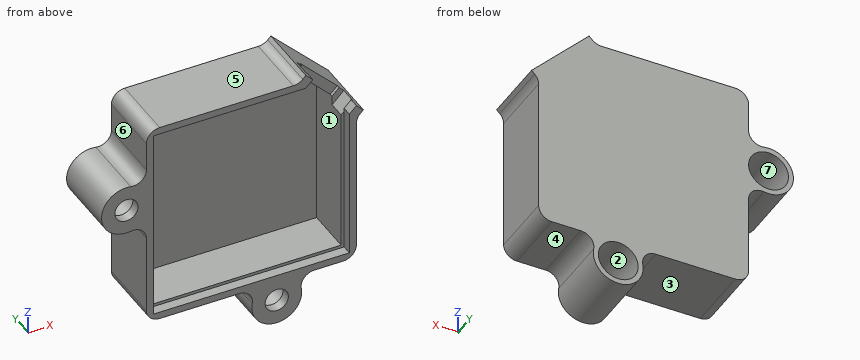
```python
from build123d import *

# Parameters (mm, degrees)
SKETCH1_W           = 31.6
SKETCH1_H           = 31.6
SKETCH1_W_2         = 28.6
SKETCH1_H_2         = 28.6
BOSS_EXTRUDE1_DEPTH = 10
SKETCH2_W           = 31.6
SKETCH2_H           = 31.6
BOSS_EXTRUDE2_DEPTH = 1.5
FILLET2_R           = 2
SKETCH3_R           = 3.75
SKETCH3_R_2         = 1.75
BOSS_EXTRUDE3_DEPTH = 10
SKETCH4_R           = 3
CUT_EXTRUDE1_DEPTH  = 8.5
CUT_EXTRUDE2_REACH  = 35.43
SKETCH6_W           = 29.5
SKETCH6_H           = 29.5
CUT_EXTRUDE3_DEPTH  = 1.5
FILLET3_R           = 2
BOSS_EXTRUDE4_DEPTH = 5.4
BOSS_EXTRUDE5_DEPTH = 4.6
BOSS_EXTRUDE6_DEPTH = 3.1
FILLET4_R           = 2
CUT_EXTRUDE6_START  = -2.5
SKETCH12_W          = 10
SKETCH12_H          = 2.6
CUT_EXTRUDE6_DEPTH  = 2.5


with BuildPart() as part:
    # Sketch1 → Boss-Extrude1 (new body)
    with BuildSketch(Plane(origin=(0, 0, 0), x_dir=(1, 0, 0), z_dir=(0, 1, 0))):
        Rectangle(SKETCH1_W, SKETCH1_H)
        Rectangle(SKETCH1_W_2, SKETCH1_H_2, mode=Mode.SUBTRACT)
    extrude(amount=BOSS_EXTRUDE1_DEPTH)

    # Sketch2 → Boss-Extrude2 (add)
    with BuildSketch(Plane.XZ.offset(-10)):
        Rectangle(SKETCH2_W, SKETCH2_H)
    extrude(amount=BOSS_EXTRUDE2_DEPTH)

    # Fillet2
    fillet2_edges = [part.edges().sort_by_distance(p)[0] for p in [
        (-15.8, 5, -15.8),
        (15.8, 5, -15.8),
        (15.8, 5, 15.8),
        (-15.8, 5, 15.8),
    ]]
    fillet(fillet2_edges, radius=FILLET2_R)

    # Sketch3 → Boss-Extrude3 (add)
    # profile 1 of 2: a face of its own
    with BuildSketch(Plane(origin=(0, 0, 0), x_dir=(1, 0, 0), z_dir=(0, 1, 0))):
        with Locations((-18.806316011, -3.821100987)):
            Circle(SKETCH3_R)
        with Locations(Location((-18.806316011, -3.821100987, 0), (0, 0, 90))):
            Circle(SKETCH3_R_2, mode=Mode.SUBTRACT)
    # profile 2 of 2: a face of its own
    with BuildSketch(Plane(origin=(0, 0, 0), x_dir=(1, 0, 0), z_dir=(0, 1, 0))):
        with Locations((3.821100987, 18.806316011)):
            Circle(SKETCH3_R)
        with Locations(Location((3.821100987, 18.806316011, 0), (0, 0, 90))):
            Circle(SKETCH3_R_2, mode=Mode.SUBTRACT)
    extrude(amount=BOSS_EXTRUDE3_DEPTH)

    # Sketch4 → Cut-Extrude1 (cut)
    with BuildSketch(Plane(origin=(0, 10, 0), x_dir=(1, 0, 0), z_dir=(0, 1, 0))):
        with Locations(Location((-18.806316011, -3.821100987, 0), (0, 0, 270))):
            Circle(SKETCH4_R)
        with Locations(Location((3.821100987, 18.806316011, 0), (0, 0, 270))):
            Circle(SKETCH4_R)
    extrude(amount=-CUT_EXTRUDE1_DEPTH, mode=Mode.SUBTRACT)

    # Sketch5 → Cut-Extrude2 (cut, up to next)
    with BuildSketch(Plane.XZ, mode=Mode.PRIVATE) as cut_extrude2_sk1:
        Polygon((14.3, 14.3), (8.643145751, 14.3), (14.3, 8.643145751), align=None)
    cut_extrude2_tool1 = extrude(cut_extrude2_sk1.sketch, amount=-CUT_EXTRUDE2_REACH, mode=Mode.PRIVATE) & part.part
    # Sketch5 → Cut-Extrude2 (cut, up to next)
    with BuildSketch(Plane.XZ, mode=Mode.PRIVATE) as cut_extrude2_sk2:
        with BuildLine():
            Line((13.8, 15.8), (7.143145751, 15.8))
            Line((7.143145751, 15.8), (8.643145751, 14.3))
            Line((8.643145751, 14.3), (14.3, 14.3))
            Line((14.3, 14.3), (14.3, 8.643145751))
            Line((14.3, 8.643145751), (15.8, 7.143145751))
            Line((15.8, 7.143145751), (15.8, 13.8))
            ThreePointArc((15.8, 13.8), (15.214213562, 15.214213562), (13.8, 15.8))
        make_face()
    cut_extrude2_tool2 = extrude(cut_extrude2_sk2.sketch, amount=-CUT_EXTRUDE2_REACH, mode=Mode.PRIVATE) & part.part
    add(cut_extrude2_tool1.solids().sort_by_distance((12.414382, 0, 12.414382))[0], mode=Mode.SUBTRACT)
    add(cut_extrude2_tool2.solids().sort_by_distance((15.127645, 0, 15.127645))[0], mode=Mode.SUBTRACT)

    # Sketch6 → Cut-Extrude3 (cut)
    with BuildSketch(Plane.XZ):
        Rectangle(SKETCH6_W, SKETCH6_H)
    extrude(amount=-CUT_EXTRUDE3_DEPTH, mode=Mode.SUBTRACT)

    # Fillet3
    fillet3_edges = [part.edges().sort_by_distance(p)[0] for p in [
        (6.062654922, 5, -15.8),
        (1.579547052, 5, -15.8),
        (-15.8, 5, 1.579547052),
        (-15.8, 5, 6.062654922),
    ]]
    fillet(fillet3_edges, radius=FILLET3_R)

    # Sketch7 → Boss-Extrude4 (add)
    with BuildSketch(Plane(origin=(0, 10, 0), x_dir=(1, 0, 0), z_dir=(0, 1, 0))):
        Polygon((8.203805922, -16.860660172), (7.143145751, -15.8), (15.8, -7.143145751), (16.860660172, -8.203805922), align=None)
    extrude(amount=-BOSS_EXTRUDE4_DEPTH)

    # Sketch8 → Boss-Extrude5 (add)
    with BuildSketch(Plane.XZ.offset(-4.6)):
        Polygon((7.143145751, 15.8), (8.193145751, 14.75), (9.253805922, 15.810660172), (8.203805922, 16.860660172), align=None)
        Polygon((16.860660172, 8.203805922), (15.810660172, 9.253805922), (14.75, 8.193145751), (15.8, 7.143145751), align=None)
    extrude(amount=BOSS_EXTRUDE5_DEPTH)

    # Sketch9 → Boss-Extrude6 (add)
    with BuildSketch(Plane.XZ.offset(-4.6)):
        Polygon((8.193145751, 14.75), (8.643145751, 14.3), (9.703805922, 15.360660172), (9.253805922, 15.810660172), align=None)
        Polygon((15.360660172, 9.703805922), (14.3, 8.643145751), (14.75, 8.193145751), (15.810660172, 9.253805922), align=None)
    extrude(amount=BOSS_EXTRUDE6_DEPTH)

    # Fillet4
    fillet4_edges = [part.edges().sort_by_distance(p)[0] for p in [
        (7.143145751, 5, 15.8),
        (15.8, 5, 7.143145751),
    ]]
    fillet(fillet4_edges, radius=FILLET4_R)

    # Sketch12 → Cut-Extrude6 (cut)
    with BuildSketch(Plane(origin=(12.532233047, 0, 12.532233047), x_dir=(0.7071067811865475, 0, -0.7071067811865477), z_dir=(0.7071067811865477, 0, 0.7071067811865475)).offset(CUT_EXTRUDE6_START)):
        with Locations((0, 2.8)):
            Rectangle(SKETCH12_W, SKETCH12_H)
    extrude(amount=CUT_EXTRUDE6_DEPTH, mode=Mode.SUBTRACT)


solid = part.part
```
Here's how the part is built. I have some questions about the finished solid (model axes, mm). Face numbers are marked on the shaded views. A direction names the side the tool comes from. Give positions to 0.01 mm unless a question says otherwise; leave off trailing zeros. Loops run counter-clockwise (first coordinate to the right, second up) from the corner with the lowest first, then second, coordinate; pieces in that order, holes last. Notation, with made-up numbers: M 8.25,-33.75 L 30.25,-33.75 A19 ccw 30.25,1.25 Z; hole C 11,-24.5 d1. An arc over 180 degrees is marked long. Put each result on its own line as item: value. Start each with the question number.
(1) I want a section at D-D on y = 2.5. State how many separate pieces and enclosed holes the cut face has, then the cut area to 3 significant figures.
(2) If we mould it in two halves opening along Z, with no side actions, what happens to the marked faces 5, 6 and 7? For each: +Z half, -Z half, draft (parallel to the pull), parting line (faces both ways), or undercut.
(3) I need wall thicknesses on line 1 along X through (y, z) = (3.5, -4); line 2 along X through (y, z) = (2.5, 6). Which ranges of each line are inside material? Lowest first, please. Write a range as [from, to].
(4) For the marked faces 1, 2, 3 and 4, which set-ups out of +Z, -Z, +X, -X, +Y, -Y let a thin tool reach every point of the face, with its end or its side?
(5) Will these pins go through, and if not, where does the flat tip stop? pin 1 Ø0.9 at (x, z) = (15, 8.5) entering from -Y; pin 2 Ø1.2 at (x, y) = (-2.5, 1) entering from -Z; pin 3 Ø1.5 at (x, y) = (6.5, 6.5) entering from +Z; pin 4 Ø4 at (x, y) = (-1, 3.5) entering from -Z.
(6) I want a section at B-B on x = 11. Please give me the cut outline in (y, z), then the cut area to 3 significant figures.
(7) I want a section at C-C on z = -9. Please give me the cut outline in (x, y), then the cut area to 4 significant figures.
(8) I want a section at A-A on z = 5. Please give me the cut outline in (x, y), then the cut area to 3 significant figures.
Answer block:
1. separate pieces: 1
1. enclosed holes: 2
1. area: 194 mm^2
2. face 5: +Z half
2. face 6: draft
2. face 7: undercut
3. line 1: [-15.8, -14.3], [14.3, 15.8]
3. line 2: [-21.86, -20.87], [-16.74, -14.3], [14.3, 15.8]
4. face 1: -Y
4. face 2: +Y
4. face 3: -Z, -X, +Y, -Y
4. face 4: -Z, +X, +Y, -Y
5. pin 1: y = 0
5. pin 2: z = -15.8
5. pin 3: z = 16.03
5. pin 4: z = -21.28
6. outline: M 0,-15.8 L 10,-15.8 L 10,14.06 L 4.6,14.06 L 4.6,11.94 L 8.5,11.94 L 8.5,-14.3 L 1.5,-14.3 L 1.5,-14.75 L 0,-14.75 Z
6. area: 65.1 mm^2
7. outline: M -15.8,0 L -14.75,0 L -14.75,1.5 L -14.3,1.5 L -14.3,8.5 L 14.3,8.5 L 14.3,1.5 L 14.75,1.5 L 14.75,0 L 15.8,0 L 15.8,10 L -15.8,10 Z
7. area: 71.55 mm^2
8. outline: M -22.37,0 L -20.1,0 L -20.1,1.5 L -21.56,1.5 L -21.56,10 L -22.37,10 Z; M -17.51,0 L -14.75,0 L -14.75,1.5 L -14.3,1.5 L -14.3,8.5 L 14.3,8.5 L 14.3,1.5 L 14.75,1.5 L 14.75,0 L 15.8,0 L 15.8,10 L -16.05,10 L -16.05,1.5 L -17.51,1.5 Z
8. area: 86.4 mm^2
